Check sheet for the modelled part. Datum: model origin and axes. Units: mm. Face numbers are marked on the shaded views. A direction names the side the tool comes from. Round coordinates to 2 decimals unless told otherwise and drop trailing zeros. Write each loop counter-clockwise with the first axis right and the second up, starting at its lowest first coordinate (ties: lowest second). Pieces come first, ordered by that corner, then holes. Notation, with made-up numbers: M -25.75,1.25 L 24.25,1.25 A14 ccw 24.25,26.25 Z; hole C 50.5,35 d2. An arc over 180 degrees is marked long. Put each result on its own line as item: value.
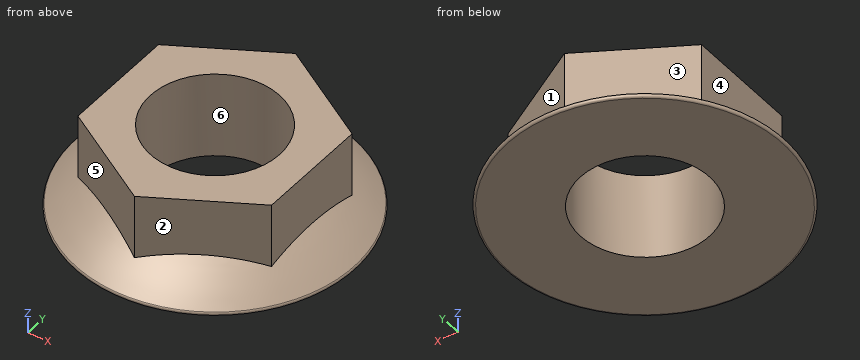
```python
from build123d import *

# Parameters (mm, degrees)
BOSS_EXTRUDE2_DEPTH = 20
SKETCH3_R           = 15
CUT_EXTRUDE1_DEPTH  = 51.060014113


with BuildPart() as part:
    # Sketch1 → Boss-Extrude2 (new body)
    with BuildSketch(Plane.XY):
        Polygon((22.5, 12.990381057), (0, 25.980762114), (-22.5, 12.990381057), (-22.5, -12.990381057), (0, -25.980762114), (22.5, -12.990381057), align=None)
    extrude(amount=BOSS_EXTRUDE2_DEPTH)

    # Sketch2 → Revolve1 (revolve)
    with BuildSketch(Plane(origin=(0, 0, 0), x_dir=(0, 0, -1), z_dir=(1, 0, 0)), mode=Mode.PRIVATE) as revolve1_sk:
        with BuildLine():
            Line((0, 0), (-12, 0))
            ThreePointArc((-12, 0), (-8.979840166, -16.995527234), (-0.900236414, -32.249684523))
            ThreePointArc((-0.900236414, -32.249684523), (-0.342073129, -32.424403945), (0, -31.95))
            Line((0, -31.95), (0, 0))
        make_face()
    revolve(revolve1_sk.sketch.rotate(Axis((0, 0, 0), (0, 0, 1)), 180), axis=Axis((0, 0, 0), (0, 0, 1)))

    # Sketch3 → Cut-Extrude1 (cut, through all)
    with BuildSketch(Plane.XY.offset(20)):
        Circle(SKETCH3_R)
    extrude(amount=-CUT_EXTRUDE1_DEPTH, mode=Mode.SUBTRACT)


solid = part.part
```
1. Scan lines: probe 1 along Y at (x, z) = (0, 6.75); probe 2 along X at (y, z) = (-12, 18.5); probe 3 along X at (y, z) = (6, 7). Record each from-to range of solid material in increasing order.
Computed values:
probe 1: y = -25.98 to -15, 15 to 25.98
probe 2: x = -22.5 to -9, 9 to 22.5
probe 3: x = -22.5 to -13.75, 13.75 to 22.5
2. Release check for a two-part mould opening along Y. For the marked faces 4, 5 and 6 record: +Y half, -Y half, draft (parallel to the pull), parting line (faces both ways), or undercut.
Computed values:
face 4: draft
face 5: -Y half
face 6: undercut
3. Depth check by flat-ended pin: pin 1 Ø12 at (y, z) = (-2.5, 11.5) entering from +X; pin 2 Ø3 at (y, z) = (6.5, 7.5) entering from -X; pin 3 Ø4.5 at (y, z) = (-4.5, 9.5) entering from -X. Enter the tip coordinate at first touch or a pass-through.
Computed values:
pin 1: stops at x = 24.89
pin 2: stops at x = -23.17
pin 3: stops at x = -22.5
4. Cross-section at A-A (z = 15). Enter the section's corners in (x, y), then the cut area to 3 significant figures.
Computed values:
outline: M -22.5,-12.99 L 0,-25.98 L 22.5,-12.99 L 22.5,12.99 L 0,25.98 L -22.5,12.99 Z; hole C 0,0 d30
area: 1,050 mm2
5. Access from +Z, -Z, +X, -X, +Y, -Y to the whole of each face (thin tool, end or side, straight path). Record for the marked faces 1, 2 and 3.
Computed values:
face 1: +Z, +X, +Y
face 2: +Z, +X, -Y
face 3: +Z, -X, +Y
